The model under review builds one solid part; all positions refer to its coordinate system, in mm. Face numbers are marked on the shaded views. A direction names the side the tool comes from. Give positions to 0.01 mm unless a question says otherwise; leave off trailing zeros. Loops run counter-clockwise (first coordinate to the right, second up) from the corner with the lowest first, then second, coordinate; pieces in that order, holes last. Notation, with made-up numbers: M -6.75,3 L 0.25,3 A14 cw 0.25,12 Z; hole C 15.5,24 d10. An arc over 180 degrees is marked long. Return JSON: item names as keys, results as strings.
```python
from build123d import *

# Parameters (mm, degrees)
BOSS_EXTRUDE1_DEPTH = 32.5
SKETCH2_R           = 5
BOSS_EXTRUDE2_DEPTH = 10


with BuildPart() as part:
    # Sketch1 → Boss-Extrude1 (new, symmetric)
    with BuildSketch(Plane(origin=(0, 0, 0), x_dir=(1, 0, 0), z_dir=(0, 1, 0))):
        with BuildLine():
            Line((-25, 4.446712056), (-26.724137931, -0.246618147))
            ThreePointArc((-26.724137931, -0.246618147), (0, -5), (26.724137931, -0.246618147))
            Line((26.724137931, -0.246618147), (25, 4.446712056))
            ThreePointArc((25, 4.446712056), (0, 0), (-25, 4.446712056))
        make_face()
    extrude(amount=BOSS_EXTRUDE1_DEPTH, both=True)

    # Sketch2 → Boss-Extrude2 (add)
    with BuildSketch(Plane.XY):
        with Locations(Location((-20, 0, 0), (0, 0, 180))):
            Circle(SKETCH2_R)
        with Locations(Location((20, 0, 0), (0, 0, 180))):
            Circle(SKETCH2_R)
    extrude(amount=BOSS_EXTRUDE2_DEPTH)


solid = part.part
```
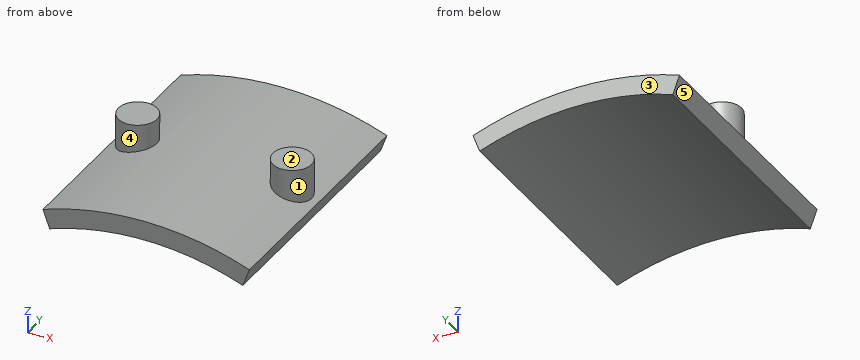
1) Tool access review of the marked faces 1 and 2: name each direction out of +Z, -Z, +X, -X, +Y, -Y from which nothing blocks a thin tool from reaching the whole face with its end or side.
From the geometry:
{"face 1": "+Z", "face 2": "+Z, +X, -X, +Y, -Y"}
2) Consider section A-A on z = 9.25. Write out the cut boundary in (x, y), then the cut area to 3 significant figures.
From the geometry:
{"outline": "C -20,0 d10; C 20,0 d10", "area": "157 mm²"}
3) Insertion check: pin 1 (1 mm diameter, centred on y = 18, z = -1, fed in from -X); pin 2 (3 mm diameter, centred on x = -18, z = 8.5, fed in from -Y); pin 3 (2 mm diameter, centred on y = 2, z = 5, fed in from +X); pin 4 (1 mm diameter, centred on x = 2, z = 7, fed in from -Y). Each pin has a flat end and moves straight along its axis. Give the tip position at first contact, or say it passes through.
From the geometry:
{"pin 1": "x = -26.45", "pin 2": "y = -4.97", "pin 3": "x = 24.9", "pin 4": "through"}
4) The part is to be moulded in two halves that separate along X. For the marked faces 3, 4 and 5, say which applies: released by +X, released by -X, zero draft, split by the parting line, or undercut.
From the geometry:
{"face 3": "zero draft", "face 4": "undercut", "face 5": "released by -X"}
5) Consider section C-C on y = 23. Write out the cut boundary in (x, z), then the cut area to 3 significant figures.
From the geometry:
{"outline": "M -26.72,0.25 L -25,-4.45 A72.5 cw 25,-4.45 L 26.72,0.25 A77.5 ccw Z", "area": "264 mm²"}
6) Consider section B-B on x = -20. Write out the cut boundary in (y, z), then the cut area to 3 significant figures.
From the geometry:
{"outline": "M -32.5,-2.81 L 32.5,-2.81 L 32.5,2.37 L 5,2.37 L 5,10 L -5,10 L -5,2.37 L -32.5,2.37 Z", "area": "413 mm²"}
7) Consider section D-D on y = -1.5. Write out the cut boundary in (x, z), then the cut area to 3 significant figures.
From the geometry:
{"outline": "M -26.72,0.25 L -25,-4.45 A72.5 cw 25,-4.45 L 26.72,0.25 A77.5 ccw 24.77,0.94 L 24.77,10 L 15.23,10 L 15.23,3.49 A77.5 ccw -15.23,3.49 L -15.23,10 L -24.77,10 L -24.77,0.94 A77.5 ccw Z", "area": "411 mm²"}
8) Wall thickness on L1, parallel to Y at x = 20, z = 5.5; L2, parallel to Y at x = -19, z = 7.5; L3, parallel to Z at x = -23, y = -25 (3 decimals): over which ranges is each line inside the solid? List them lowest first. Write a range as from..to.
From the geometry:
{"L1": "-5..5", "L2": "-4.9..4.9", "L3": "-3.745..1.508"}
